The listing builds one solid part. Answer for the finished solid, in the listing's coordinates (mm). Face numbers are marked on the shaded views. A direction names the side the tool comes from. Round coordinates to 2 decimals unless told otherwise and drop trailing zeros. Loops run counter-clockwise (first coordinate to the right, second up) from the corner with the lowest first, then second, coordinate; pieces in that order, holes last. Notation, with made-up numbers: M -29,1 L -12,1 A21 ccw -12,6 Z; hole C 22,-33.75 d5. An arc over 180 degrees is marked long. Put each result on its own line as item: value. Start each with the question number.
(1) Which of the six approach directions +Z, -Z, +X, -X, +Y, -Y give full straight-line access (tool end or side, diameter ignored) to the marked faces 1 and 2?
(2) Determine the mould class of the marked faces 3, 4 and 5 for opening direction X: released by +X, released by -X, zero draft, split by the parting line, or undercut.
(3) Section D-D, the plane z = 4.25 is taken. Determine the outline of the cut face in (x, y).
(4) Section A-A, the plane y = -0.5 is taken. Determine the outline of the cut face in (x, z).
(5) Section C-C, the plane z = 13.75 is taken. Determine the outline of the cut face in (x, y).
(6) Flat-ended cylindrical pins translate along their axes: P1, Ø1.6, axis at x = 3, z = -2, coming from the -Y side; P2, Ø1, axis at x = 1, z = 8, coming from the +Y side; P3, Ø2, axis at x = 2.5, z = -2, coming from the +Y side. Find the tip coordinate at first contact, or state that the pin passes through.
(7) Straight lines are drawn through the part: line 1 (Y direction, x = 4.75, z = -0.75); line 2 (Z direction, x = 6.25, y = 0.25); line 3 (Z direction, x = 2.75, y = 3.5). For each, find the intervals that lie inside material, in ascending order.
(8) Section B-B, the plane x = 3.5 is taken. Determine the outline of the cut face in (y, z).
```python
from build123d import *

# Parameters (mm, degrees)
F0_R     = 4
F1_DEPTH = 12
F2_R     = 3
F2_R_2   = 2.287122
F3_DEPTH = 5
F4_W     = 0.61053
F4_H     = 1.999993
F4_W_2   = 0.53819
F4_H_2   = 1.892356
F4_W_3   = 2.00924
F4_H_3   = 0.50231
F5_DEPTH = 3


with BuildPart() as f1:
    # F0 (on Top) → F1 (new body)
    with BuildSketch(Plane.XY):
        with Locations((2.705152, 0.901718)):
            Circle(F0_R)
    extrude(amount=F1_DEPTH)

    # F2 (on face) → F3 (join)
    with BuildSketch(Plane.XY.offset(12)):
        with Locations((2.705152, 0.901718)):
            Circle(F2_R)
        with Locations((2.705152, 0.901718)):
            Circle(F2_R_2, mode=Mode.SUBTRACT)
    extrude(amount=F3_DEPTH)

    # F4 (on face) → F5 (join)
    with BuildSketch(Plane(origin=(0, 0, 0), x_dir=(1, 0, 0), z_dir=(0, 0, -1))):
        with Locations((0.305265, -0.999996)):
            Rectangle(F4_W, F4_H)
        with Locations((4.969864, -0.946178)):
            Rectangle(F4_W_2, F4_H_2)
        with Locations((2.763287, 1.229143)):
            Rectangle(F4_W_3, F4_H_3)
    extrude(amount=F5_DEPTH)


solid = f1.part
```
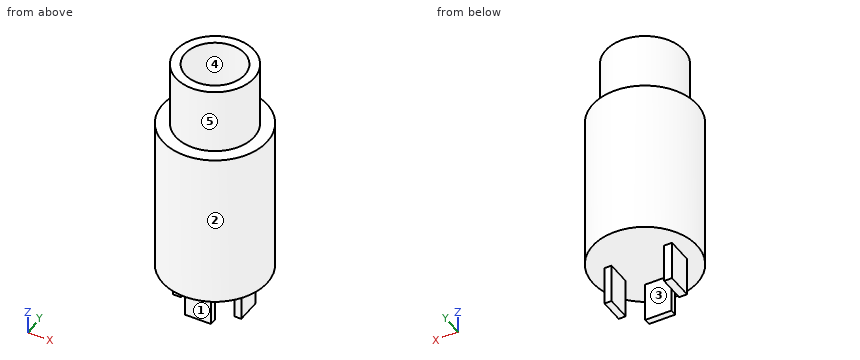
Recorded:
1. face 1: -Z, +X, -X, -Y
1. face 2: +Z, -Z
2. face 3: zero draft
2. face 4: undercut
2. face 5: split by the parting line
3. outline: C 2.71,0.9 d8
4. outline: M -1.04,0 L 6.45,0 L 6.45,12 L 5.36,12 L 5.36,17 L 4.51,17 L 4.51,12 L 0.9,12 L 0.9,17 L 0.05,17 L 0.05,12 L -1.04,12 Z
5. outline: C 2.71,0.9 d6; hole C 2.71,0.9 d4.57
6. P1: stops at y = -1.48
6. P2: stops at y = 4.72
6. P3: stops at y = -0.98
7. line 1: y = 0 to 1.89
7. line 2: z = 0 to 12
7. line 3: z = 0 to 17
8. outline: M -3.02,0 L -1.48,0 L -1.48,-3 L -0.98,-3 L -0.98,0 L 4.82,0 L 4.82,12 L 3.79,12 L 3.79,17 L 3.05,17 L 3.05,12 L -1.24,12 L -1.24,17 L -1.99,17 L -1.99,12 L -3.02,12 Z
